from build123d import *

# Parameters (mm, degrees)
F0_W      = 20
F0_H      = 20
F0_R      = 8.65
F1_DEPTH  = 20
F2_W      = 20
F2_H      = 20
F3_DEPTH  = 15
F4_R      = 4.75
F5_DEPTH  = 8
F6_R      = 2.075
F7_DEPTH  = 11
F9_DEPTH  = 25.3
F10_W     = 6
F10_H     = 2
F11_DEPTH = 3.5
F12_R     = 2.15
F13_DEPTH = 5.23
F14_R     = 1.65
F15_DEPTH = 6.34
F16_R     = 3.5
F17_DEPTH = 31.8
F18_R     = 5
F20_W     = 10
F20_H     = 16
F21_DEPTH = 9.7
F22_DEPTH = 5
F23_R     = 2.15
F24_DEPTH = 12.5
F25_R     = 5


with BuildPart() as f1:
    # F0 (on Front) → F1 (new body)
    with BuildSketch(Plane.XZ):
        Rectangle(F0_W, F0_H)
        Circle(F0_R, mode=Mode.SUBTRACT)
    extrude(amount=F1_DEPTH)

    # F2 (on Front) → F3 (join)
    with BuildSketch(Plane.XZ):
        Rectangle(F2_W, F2_H)
    extrude(amount=-F3_DEPTH)

    # F4 (on Front) → F5 (cut)
    with BuildSketch(Plane.XZ):
        Circle(F4_R)
    extrude(amount=-F5_DEPTH, mode=Mode.SUBTRACT)

    # F6 (on Front) → F7 (cut)
    with BuildSketch(Plane.XZ):
        Circle(F6_R)
    extrude(amount=-F7_DEPTH, mode=Mode.SUBTRACT)

    # F8 (on Front) → F9 (cut, symmetric)
    with BuildSketch(Plane.XZ):
        Polygon((4.25, 0), (-10, 0.75), (-10, -0.75), align=None)
    extrude(amount=F9_DEPTH, both=True, mode=Mode.SUBTRACT)

    # F10 (on Front) → F11 (join, symmetric)
    with BuildSketch(Plane.XZ):
        with Locations((-13, 1.75)):
            Rectangle(F10_W, F10_H)
        with Locations((-13, -1.75)):
            Rectangle(F10_W, F10_H)
    extrude(amount=F11_DEPTH, both=True)

    # F12 (on Top) → F13 (cut, symmetric)
    with BuildSketch(Plane.XY):
        with Locations((-13, 0)):
            Circle(F12_R)
    extrude(amount=F13_DEPTH, both=True, mode=Mode.SUBTRACT)

    # F14 (on Top) → F15 (cut)
    with BuildSketch(Plane.XY):
        with Locations((-13, 0)):
            Circle(F14_R)
    extrude(amount=-F15_DEPTH, mode=Mode.SUBTRACT)

    # F16 (on Front) → F17 (cut)
    with BuildSketch(Plane.XZ):
        Circle(F16_R)
    extrude(amount=-F17_DEPTH, mode=Mode.SUBTRACT)

    # F18
    f18_edges = [f1.edges().sort_by_distance(p)[0] for p in [
        (-10, -2.5, -10),
        (-10, -2.5, 10),
    ]]
    fillet(f18_edges, radius=F18_R)

    # F20 (on Right) → F21 (join)
    with BuildSketch(Plane.YZ):
        with Locations((20, 0)):
            Rectangle(F20_W, F20_H)
    extrude(amount=F21_DEPTH)

    # F20 (on Right) → F22 (cut)
    with BuildSketch(Plane.YZ):
        with Locations((20, 0)):
            Rectangle(F20_W, F20_H)
    extrude(amount=F22_DEPTH, mode=Mode.SUBTRACT)

    # F23 (on face) → F24 (cut, symmetric)
    with BuildSketch(Plane.YZ):
        with Locations((21, 4)):
            Circle(F23_R)
        with Locations((21, -4)):
            Circle(F23_R)
    extrude(amount=F24_DEPTH, both=True, mode=Mode.SUBTRACT)

    # F25
    f25_edges = [f1.edges().sort_by_distance(p)[0] for p in [
        (7.35, 25, -8),
        (7.35, 25, 8),
    ]]
    fillet(f25_edges, radius=F25_R)


solid = f1.part
Geometry: final body of the model. Coordinates: model frame, mm. A direction names the side the tool comes from. Give positions to 0.01 mm unless a question says otherwise; leave off trailing zeros. Loops run counter-clockwise (first coordinate to the right, second up) from the corner with the lowest first, then second, coordinate; pieces in that order, holes last. Notation, with made-up numbers: (-23.5, -18) -> (20.5, -18) arc R20 ccw to (20.5, 12) -> close; hole circle Ø10 at (-15.5, -29.5). An arc over 180 degrees is marked (long way). Put each result on its own line as item: value.
1. Ray query, line 1 along Y through (x, z) = (-13, 1.3); line 2 along Z through (x, y) = (7.55, 21); line 3 along X through (y, z) = (-2, 0). Return the intervals inside material, ascending. Write a range as [from, to].
Taken from the geometry:
line 1: y = [-3.5, -2.15], [2.15, 3.5]
line 2: z = [-7.9, -6.15], [-1.85, 1.85], [6.15, 7.9]
line 3: x = [8.65, 10]
2. Cut plane C-C (y = 9). Return the cut outline in (x, z), plus the area to 3 significant figures.
Taken from the geometry:
outline: (-10, -5) arc R5 ccw to (-5, -10) -> (10, -10) -> (10, 10) -> (-5, 10) arc R5 ccw to (-10, 5) -> (-10, 0.75) -> (-3.48, 0.41) arc R3.5 cw to (3.5, 0.04) -> (4.25, 0) -> (3.5, -0.04) arc R3.5 cw to (-3.48, -0.41) -> (-10, -0.75) -> close
area: 343 mm2
3. Cut plane B-B (x = 0). Return the cut outline in (y, z), plus the area to 3 significant figures.
Taken from the geometry:
outline: (-20, -10) -> (15, -10) -> (15, -3.5) -> (8, -3.5) -> (8, -4.75) -> (0, -4.75) -> (0, -8.65) -> (-20, -8.65) -> close; (-20, 8.65) -> (0, 8.65) -> (0, 4.75) -> (8, 4.75) -> (8, 3.5) -> (15, 3.5) -> (15, 10) -> (-20, 10) -> close
area: 229 mm2
4. Cut plane D-D (z = 4). Return the cut outline in (x, y), plus the area to 3 significant figures.
Taken from the geometry:
outline: (-10, -20) -> (-7.67, -20) -> (-7.67, 0) -> (-2.56, 0) -> (-2.56, 8) -> (2.56, 8) -> (2.56, 0) -> (7.67, 0) -> (7.67, -20) -> (10, -20) -> (10, 15) -> (9.7, 15) -> (9.7, 18.85) -> (5, 18.85) -> (5, 15) -> (-10, 15) -> close; (5, 23.15) -> (9.7, 23.15) -> (9.7, 24.9) -> (5, 24.9) -> close
area: 379 mm2
5. Pull-direction query (Y, two-part tool) for faces 4 (the cylindrical face through (7.32, 21.99, 2.09)), 5 (the flat face through (-16, 0, 2)), 6 (the flat face through (4, 0, -4)); classes: released by +Y, released by -Y, zero draft, split by the parting line, or undercut.
Taken from the geometry:
face 4: undercut
face 5: zero draft
face 6: released by -Y
6. Cut plane A-A (x = -13). Return the cut outline in (y, z).
Taken from the geometry:
outline: (-3.5, -2.75) -> (-2.15, -2.75) -> (-2.15, -0.75) -> (-3.5, -0.75) -> close; (-3.5, 0.75) -> (-2.15, 0.75) -> (-2.15, 2.75) -> (-3.5, 2.75) -> close; (2.15, -2.75) -> (3.5, -2.75) -> (3.5, -0.75) -> (2.15, -0.75) -> close; (2.15, 0.75) -> (3.5, 0.75) -> (3.5, 2.75) -> (2.15, 2.75) -> close
7. Set-up query: faces 1 (the flat face through (-13, 2.4, 2.75)), 2 (the cylindrical face through (0.1, 11.5, -3.5)), 3 (the flat face through (-13, -2.4, -2.75)). Return all of +Z, -Z, +X, -X, +Y, -Y with unobstructed straight access to the full face (end or side cutting, diameter ignored); none if empty.
Taken from the geometry:
face 1: +Z, -X, +Y, -Y
face 2: +Y, -Y
face 3: -Z, -X, +Y, -Y
8. Pin query (flat end, axial travel): P1, Ø2.5, axis at x = 8, y = 16.5, coming from the +Z side; P2, Ø5, axis at y = 21, z = -4, coming from the +X side; P3, Ø3, axis at x = -13, y = 1.5, coming from the -Z side; P4, Ø3.5, axis at x = -13, y = 0, coming from the -Z side. Return the tip coordinate at first contact, or that it passes through.
Taken from the geometry:
P1: stops at z = 8
P2: stops at x = 9.7
P3: stops at z = -2.75
P4: passes through
